Input: part model. Units: mm. Frame: model coordinates. A direction names the side the tool comes from. Coordinates: 2 decimals unless noted, no trailing zeros. Order: outer loops, then holes, each group sorted by start corner. A loop starts at its lowest first (then second) coordinate and runs counter-clockwise, first axis right, second up. Notation, with made-up numbers: (59.5, -5) -> (95.5, -5) arc R23 cw to (95.5, 30) -> close; hole circle Ø4 at (-14, 5.5). An arc over 180 degrees is marked (long way). Use one line per item in the form item = value. Start each with the question number.
1) Draft query along Z for faces 1 (the flat face through (34, 17, 5)), 2 (the cylindrical face through (16.93, 2.47, 3.39)), 3 (the flat face through (17, 21, 10)). Return one class per face: pulls with the +Z half, pulls with the -Z half, needs draft (parallel to the pull), parting line crosses it, or undercut.
2) Section query D-D on z = 5. Count the separate pieces of the cut face and the enclosed holes in it, then the cut area to 3 significant figures.
3) Pin query (flat end, axial travel): pin 1 (1.5 mm diameter, centred on y = 6, z = 2.5, fed in from -X); pin 2 (5 mm diameter, centred on x = 31, z = 5.5, fed in from +Y). Return the tip coordinate at first contact, or that it passes through.
4) Access query for faces 4 (the flat face through (12, 25, 5)), 5 (the flat face through (22, 25, 5)), 6 (the flat face through (25, 12, 5)), 7 (the flat face through (9, 12, 5)). Directions: +Z, -Z, +X, -X, +Y, -Y. A direction counts if a zero-diameter tool reaches every point of the face in a straight line with its end or side. Return the directions, or none.
5) Section query C-C on z = 1.5. Output: boundary loops of the cut face in (x, y).
6) Section query A-A on x = 17. Output: boundary loops of the cut face in (y, z), then the cut area to 3 significant figures.
7) Ray query, line 1 along Z through (x, y) = (5, 18); line 2 along X through (y, z) = (18.5, 5); line 3 along X through (y, z) = (16, 2.25). Return the intervals inside material, ascending.
Autodesk Inventor part; units mm, degrees
ref_plane "YZ Plane" through (0, 0, 0) normal (1, 0, 0) x (0, 1, 0)
ref_plane "XZ Plane" through (0, 0, 0) normal (0, 1, 0) x (-1, 0, 0)
ref_plane "XY Plane" through (0, 0, 0) normal (0, 0, 1) x (1, 0, 0)
sketch "スケッチ1" plane through (0, 0, 0) normal (0, 0, 1) x (1, 0, 0)
  line L0 (0, 0) -> (34, 0)
  line L1 (34, 0) -> (34, 34)
  line L2 (34, 34) -> (0, 34)
  line L3 (0, 34) -> (0, 0)
  dimension "d0" = 34
  dimension "d1" = 34
extrude "押し出し1" add sketch "スケッチ1" along normal blind 10
sketch "スケッチ2" plane through (0, 0, 10) normal (0, 0, 1) x (1, 0, 0)
  line L0 (34, 34) -> (0, 34)
  line L1 (34, 34) -> (22, 34)
  line L2 (22, 34) -> (22, 22)
  line L3 (22, 22) -> (34, 22)
  line L4 (34, 22) -> (34, 34)
  point P0 (0, 0)
  point P1 (22, 34)
  dimension "d4" = 12
  dimension "d5" = 12
extrude "押し出し2" cut sketch "スケッチ2" against normal blind 10
sketch "スケッチ3" plane through (0, 0, 10) normal (0, 0, 1) x (1, 0, 0)
  line L0 (0, 34) -> (12, 34)
  line L1 (12, 34) -> (12, 22)
  line L2 (12, 22) -> (0, 22)
  line L3 (0, 22) -> (0, 34)
  line L4 (0, 0) -> (34, 0)
  line L5 (0, 0) -> (12, 0)
  line L6 (12, 0) -> (12, 12)
  line L7 (12, 12) -> (0, 12)
  line L8 (0, 12) -> (0, 0)
  line L9 (34, 0) -> (22, 0)
  line L10 (22, 0) -> (22, 12)
  line L11 (22, 12) -> (34, 12)
  line L12 (34, 12) -> (34, 0)
  point P0 (22, 0)
  dimension "d8" = 12
  dimension "d9" = 12
  dimension "d10" = 12
  dimension "d11" = 12
  dimension "d12" = 12
  dimension "d13" = 12
extrude "押し出し3" cut sketch "スケッチ3" against normal blind 10
sketch "スケッチ4" plane through (22, 22, 10) normal (1, 0, 0) x (0, 0, -1)
  line L0 (0, 12) -> (10, 12)
  line L1 (10, 12) -> (10, 0)
  line L2 (10, -10) -> (10, -22)
  line L3 (10, -22) -> (0, -22)
  point P0 (5, 7)
  point P1 (5, -17)
  dimension "d16" = 5
  dimension "d17" = 5
  dimension "d18" = 5
  dimension "d19" = 5
hole "穴1" at (22, 29, 5) at (22, 5, 5) direction (-1, 0, 0) diameter 6 end through all
sketch "スケッチ5" plane through (0, 22, 10) normal (0, 1, 0) x (1, 0, 0)
  line L0 (0, 10) -> (12, 10)
  line L1 (0, 0) -> (0, 10)
  line L2 (22, 10) -> (34, 10)
  line L3 (34, 10) -> (34, 0)
  point P0 (5, 5)
  point P1 (29, 5)
  dimension "d27" = 5
  dimension "d28" = 5
  dimension "d29" = 5
  dimension "d30" = 5
hole "穴2" at (5, 22, 5) at (29, 22, 5) direction (0, -1, 0) diameter 6 end through all
sketch "スケッチ6" plane through (0, 0, 10) normal (0, 0, 1) x (1, 0, 0)
  line L0 (34, 12) -> (34, 22)
  line L1 (22, 34) -> (12, 34)
  point P0 (0, 0)
  point P1 (17, 17)
  dimension "d38" = 17
  dimension "d39" = 17
hole "穴3" at (17, 17, 10) direction (0, 0, -1) diameter 2.459 end through all
properties part number "シリンダ先端パーツ"
Answers below:
q1.face_1 = needs draft
q1.face_2 = undercut
q1.face_3 = pulls with the +Z half
q2.separate_pieces = 5
q2.enclosed_holes = 1
q2.area = 335 mm^2
q3.pin_1 = 12
q3.pin_2 = 22
q4.face_4 = +Z, -Z, -X, +Y
q4.face_5 = +Z, -Z, +X, +Y
q4.face_6 = +Z, -Z, +X, -Y
q4.face_7 = +Z, -Z, -X, -Y
q5.outline = (0, 12) -> (12, 12) -> (12, 0) -> (22, 0) -> (22, 12) -> (34, 12) -> (34, 22) -> (22, 22) -> (22, 34) -> (12, 34) -> (12, 22) -> (0, 22) -> close; hole circle Ø2.46 at (17, 17)
q6.outline = (0, 0) -> (15.77, 0) -> (15.77, 10) -> (0, 10) -> close; (18.23, 0) -> (34, 0) -> (34, 10) -> (18.23, 10) -> close; hole circle Ø6 at (5, 5); hole circle Ø6 at (29, 5)
q6.area = 259 mm^2
q7.line_1 = 0 to 2, 8 to 10
q7.line_2 = 0 to 2, 8 to 26, 32 to 34
q7.line_3 = 0 to 3.8, 6.2 to 16.28, 17.72 to 27.8, 30.2 to 34
